Source: CAD feature listing. Evaluate the final solid. Frame: model axes, mm. Give positions to 0.01 mm unless a question says otherwise; leave off trailing zeros. Order: outer loops, then holes, each group sorted by start corner. A loop starts at its lowest first (then second) coordinate and runs counter-clockwise, first axis right, second up.
```python
from build123d import *

# Parameters (mm, degrees)
F0_R     = 9.5
F1_DEPTH = 13


# Not quite as in the source:
# - a fillet or chamfer that OpenCascade refuses, or shapes differently, is made with other operations: its cross-section is extruded or revolved along the edge and cut away or added


with BuildPart() as f1:
    # F0 (on Top) → F1 (new body)
    with BuildSketch(Plane.XY):
        Polygon((6.024763409, 12.5105501281), (-6.024763409, 12.5105501281), (-13.5375204973, 3.0898507129), (-10.856248536, -8.6575693106), (0, -13.885663061), (10.856248536, -8.6575693106), (13.5375204973, 3.0898507129), align=None)
        Circle(F0_R, mode=Mode.SUBTRACT)
    extrude(amount=F1_DEPTH)

    # F2: fillet of radius 6 on 3 edges, made by hand

    # F2_s1 → F2_t2 (revolve, cut)
    with BuildSketch(Plane.XZ):
        with BuildLine():
            ThreePointArc((9.5, 6), (11.2573593129, 1.7573593129), (15.5, 0))
            Line((15.5, 0), (9.5, 0))
            Line((9.5, 0), (9.5, 6))
        make_face()
    revolve(axis=Axis((0, 0, 0), (0, 0, 1)), mode=Mode.SUBTRACT)

    # F2_s3 → F2_t4 (revolve, cut)
    with BuildSketch(Plane.XZ):
        with BuildLine():
            ThreePointArc((9.5, 7), (11.2573593129, 11.2426406871), (15.5, 13))
            Line((15.5, 13), (9.5, 13))
            Line((9.5, 13), (9.5, 7))
        make_face()
    revolve(axis=Axis((0, 0, 13), (0, 0, 1)), mode=Mode.SUBTRACT)


solid = f1.part
```
1) Material intervals for L1, parallel to Y at x = 0, z = 6.4; L2, parallel to X at y = 4.75, z = 5.5; L3, parallel to Y at x = -4, z = 5, sorted ascending.
Report:
L1: y = -13.89 to -9.5, 9.5 to 12.51
L2: x = -12.21 to -8.25, 8.25 to 12.21
L3: y = -11.96 to -8.71, 8.71 to 12.51
2) Section query B-B, the plane z = 4. Return the cut outline in (x, y), and give its area (3 significant figures).
Report:
outline: (-13.54, 3.09) - (-10.86, -8.66) - (0, -13.89) - (10.86, -8.66) - (13.54, 3.09) - (6.02, 12.51) - (-6.02, 12.51) - close; hole circle Ø19.69 at (0, 0)
area: 223 mm2
3) Section query C-C, the plane z = 9.5. Return the cut outline in (x, y), and give its area (3 significant figures).
Report:
outline: (-13.54, 3.09) - (-10.86, -8.66) - (0, -13.89) - (10.86, -8.66) - (13.54, 3.09) - (6.02, 12.51) - (-6.02, 12.51) - close; hole circle Ø20.09 at (0, 0)
area: 211 mm2
4) Section query A-A, the plane y = 0. Return the cut outline in (x, z), and give its area (3 significant figures).
Report:
outline: (-12.83, 0.63) arc R6 ccw to (-9.5, 6) - (-9.5, 7) arc R6 ccw to (-12.83, 12.37) - close; (9.5, 6) arc R6 ccw to (12.83, 0.63) - (12.83, 12.37) arc R6 ccw to (9.5, 7) - close
area: 57.9 mm2
5) Pin query (flat end, axial travel): pin 1 (1 mm diameter, centred on y = -11, z = 2, fed in from +X); pin 2 (1.5 mm diameter, centred on y = -4.5, z = 6, fed in from +X); pin 3 (2 mm diameter, centred on x = 7, z = 3, fed in from -Y); pin 4 (15 mm diameter, centred on x = 0, y = 0, fed in from +Z). Return the tip coordinate at first contact, or that it passes through.
Report:
pin 1: stops at x = 7.03
pin 2: stops at x = 11.98
pin 3: stops at y = -11
pin 4: passes through
